Verification items for the finished model (mm, model axes). A direction names the side the tool comes from. Round coordinates to 2 decimals unless told otherwise and drop trailing zeros. Order: outer loops, then holes, each group sorted by start corner. A loop starts at its lowest first (then second) coordinate and runs counter-clockwise, first axis right, second up. Notation, with made-up numbers: M 76.5,88.25 L 80.5,88.25 A36 ccw 80.5,124.25 Z; hole C 37,-34.5 d7. An arc over 180 degrees is marked long. Return JSON: item names as keys, results as strings. Group by question number.
from build123d import *

# Parameters (mm, degrees)
F1_DEPTH       = 12.7
F2_T           = -2.54
F4_D           = 0.25
F4_CBORE_D     = 12.7
F4_CBORE_DEPTH = 0


with BuildPart() as f1:
    # F0 (on Front) → F1 (new body)
    with BuildSketch(Plane.XZ):
        with BuildLine():
            Line((30.532771, 96.341363), (-30.200021, 96.341363))
            ThreePointArc((-30.200021, 96.341363), (-38.122194, 93.059891), (-41.403666, 85.137717))
            Line((-41.403666, 85.137717), (-41.403666, -71.078406))
            ThreePointArc((-41.403666, -71.078406), (-38.122194, -79.00058), (-30.200021, -82.282051))
            Line((-30.200021, -82.282051), (30.532771, -82.282051))
            ThreePointArc((30.532771, -82.282051), (38.454945, -79.00058), (41.736417, -71.078406))
            Line((41.736417, -71.078406), (41.736417, 85.137717))
            ThreePointArc((41.736417, 85.137717), (38.454945, 93.059891), (30.532771, 96.341363))
        make_face()
    extrude(amount=F1_DEPTH)

    # F2
    f2_openings = [f1.faces().sort_by_distance(p)[0] for p in [
        (0.166375, -12.7, 7.029656),
    ]]
    offset(amount=F2_T, openings=f2_openings)

    # F4 (through all)
    with Locations(Plane(origin=(0, 0, -82.282051), x_dir=(1, 0, 0), z_dir=(0, 0, -1))):
        with Locations((-25.25001, 5.65)):
            CounterBoreHole(F4_D / 2, F4_CBORE_D / 2, F4_CBORE_DEPTH)


solid = f1.part
1. Draft check along Z on faces 3 (the face through (-41.404, -6, 8)), 4 (the face through (-38.03, -6.26, 93.15)), 5 (the face through (39.196, -8, 6)). Enter one of: +Z half, -Z half, draft (parallel to the pull), parting line (faces both ways), or undercut.
2. Thickness scan on line 1 along X through (y, z) = (-11.75, -32); line 2 along Z through (x, y) = (22.5, -7.75); line 3 along Y through (x, z) = (21, 32). Record the ranges inside material, lowest first. Write a range as from..to.
3. Access from +Z, -Z, +X, -X, +Y, -Y to the whole of each face (thin tool, end or side, straight path). Record for faces 1 (the face through (-38.21, -6.26, -78.91)), 2 (the face through (1, -8, 93.801)).
4. Cross-section at A-A (x = -8). Enter the section's corners in (y, z).
5. Go/stop test with flat-tipped pins: pin 1 (1.5 mm diameter, centred on x = -7, z = -59.5, fed in from -Y); pin 2 (4 mm diameter, centred on x = -30, z = 76, fed in from +Y). Record where each tip stops, or that it passes through.
6. Cross-section at B-B (z = 42.5). Enter the section's corners in (x, y).
7. Cross-section at C-C (y = -8.25). Enter the section's corners in (x, z).
Computed:
{
 "1": {"face 3": "draft", "face 4": "+Z half", "face 5": "undercut"},
 "2": {"line 1": "x = -41.4..-38.86, 39.2..41.74", "line 2": "z = -82.28..-79.74, 93.8..96.34", "line 3": "y = -2.54..0"},
 "3": {"face 1": "-Z, -X, +Y, -Y", "face 2": "-Y"},
 "4": {"outline": "M -12.7,-82.28 L 0,-82.28 L 0,96.34 L -12.7,96.34 L -12.7,93.8 L -2.54,93.8 L -2.54,-79.74 L -12.7,-79.74 Z"},
 "5": {"pin 1": "stops at y = -2.54", "pin 2": "stops at y = 0"},
 "6": {"outline": "M -41.4,-12.7 L -38.86,-12.7 L -38.86,-2.54 L 39.2,-2.54 L 39.2,-12.7 L 41.74,-12.7 L 41.74,0 L -41.4,0 Z"},
 "7": {"outline": "M -41.4,-71.08 A11.2 ccw -30.2,-82.28 L 30.53,-82.28 A11.2 ccw 41.74,-71.08 L 41.74,85.14 A11.2 ccw 30.53,96.34 L -30.2,96.34 A11.2 ccw -41.4,85.14 Z; hole M -38.86,-71.08 A8.66 ccw -30.2,-79.74 L 30.53,-79.74 A8.66 ccw 39.2,-71.08 L 39.2,85.14 A8.66 ccw 30.53,93.8 L -30.2,93.8 A8.66 ccw -38.86,85.14 Z"}
}
